Work out the finished part from the listing and answer in its coordinate system (mm). Face numbers are marked on the shaded views. A direction names the side the tool comes from. Coordinates: 2 decimals unless noted, no trailing zeros. Loops run counter-clockwise (first coordinate to the right, second up) from the corner with the lowest first, then second, coordinate; pieces in that order, holes last. Notation, with made-up numbers: (6, 79.5) -> (40, 79.5) arc R13 cw to (40, 95.5) -> close; hole circle Ø7 at (-25.5, 15.25). An arc over 180 degrees is marked (long way). Use a Markdown table: item, result.
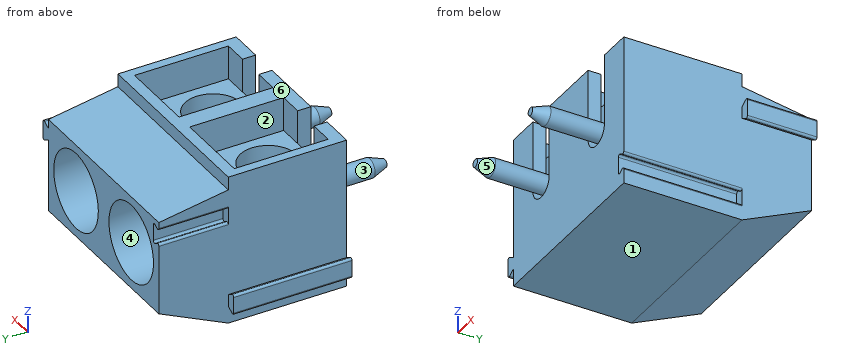
from build123d import *

# Parameters (mm, degrees)
BOSS_EXTRUDE1_DEPTH      = 10.16
SKETCH2_W                = 4.1
SKETCH2_H                = 5
CUT_EXTRUDE1_DEPTH       = 5.8
SKETCH3_W                = 4.1
SKETCH3_H                = 5
CUT_EXTRUDE2_DEPTH       = 5.8
CUT_EXTRUDE3_DEPTH       = 1
CUT_EXTRUDE4_DEPTH       = 1
BOSS_EXTRUDE2_DEPTH      = 2
BOSS_EXTRUDE2_DEPTH_BACK = 2
SKETCH6_W                = 4.1
SKETCH6_H                = 4.7
SKETCH6_R                = 1.5
BOSS_EXTRUDE3_DEPTH      = 2
BOSS_EXTRUDE3_DEPTH_BACK = 2
SKETCH7_W                = 4.1
SKETCH7_H                = 4.7
SKETCH7_R                = 1.5
SKETCH10_W               = 2.05
SKETCH10_H               = 2
SKETCH11_W               = 2.05
SKETCH11_H               = 2
BOSS_EXTRUDE4_DEPTH      = 6.3
CUT_EXTRUDE5_DEPTH       = 6.3
CUT_EXTRUDE6_DEPTH       = 3.7
BOSS_EXTRUDE5_DEPTH      = 3.7


with BuildPart() as part:
    # Sketch1 → Boss-Extrude1 (new body)
    with BuildSketch(Plane(origin=(0, 0, 0), x_dir=(0, 0, -1), z_dir=(1, 0, 0))):
        Polygon((-8, 0), (0, 0), (0, 6.3), (-1.7, 10), (-6.7, 10), (-7.3, 6.3), (-8, 6.3), align=None)
    extrude(amount=BOSS_EXTRUDE1_DEPTH)

    # Sketch2 → Cut-Extrude1 (cut)
    with BuildSketch(Plane.XY.offset(8)):
        with Locations((2.54, 3.2)):
            Rectangle(SKETCH2_W, SKETCH2_H)
    extrude(amount=-CUT_EXTRUDE1_DEPTH, mode=Mode.SUBTRACT)

    # Sketch3 → Cut-Extrude2 (cut)
    with BuildSketch(Plane.XY.offset(8)):
        with Locations((7.62, 3.2)):
            Rectangle(SKETCH3_W, SKETCH3_H)
    extrude(amount=-CUT_EXTRUDE2_DEPTH, mode=Mode.SUBTRACT)

    # Sketch4 → Cut-Extrude3 (cut)
    with BuildSketch(Plane(origin=(0, 0, 0), x_dir=(-1, 0, 0), z_dir=(0, 1, 0))):
        with BuildLine():
            Line((-1.79, 4.2), (-1.79, 8))
            Line((-1.79, 8), (-3.29, 8))
            Line((-3.29, 8), (-3.29, 4.2))
            ThreePointArc((-3.29, 4.2), (-2.54, 3.45), (-1.79, 4.2))
        make_face()
    extrude(amount=CUT_EXTRUDE3_DEPTH, mode=Mode.SUBTRACT)

    # Sketch5 → Cut-Extrude4 (cut)
    with BuildSketch(Plane(origin=(0, 0, 0), x_dir=(-1, 0, 0), z_dir=(0, 1, 0))):
        with BuildLine():
            Line((-6.87, 4.2), (-6.87, 8))
            Line((-6.87, 8), (-8.37, 8))
            Line((-8.37, 8), (-8.37, 4.2))
            ThreePointArc((-8.37, 4.2), (-7.62, 3.45), (-6.87, 4.2))
        make_face()
    extrude(amount=CUT_EXTRUDE4_DEPTH, mode=Mode.SUBTRACT)

    # Sketch6 → Boss-Extrude2 (add, two sides: drawn at the far end of the back side and taken through both)
    with BuildSketch(Plane.XY.offset(4.2).offset(-BOSS_EXTRUDE2_DEPTH_BACK)):
        with Locations((2.54, 3.05)):
            Rectangle(SKETCH6_W, SKETCH6_H)
        with Locations((2.54, 2.7)):
            Circle(SKETCH6_R, mode=Mode.SUBTRACT)
    extrude(amount=BOSS_EXTRUDE2_DEPTH + BOSS_EXTRUDE2_DEPTH_BACK)

    # Sketch7 → Boss-Extrude3 (add, two sides: drawn at the far end of the back side and taken through both)
    with BuildSketch(Plane.XY.offset(4.2).offset(-BOSS_EXTRUDE3_DEPTH_BACK)):
        with Locations((7.62, 3.05)):
            Rectangle(SKETCH7_W, SKETCH7_H)
        with Locations((7.62, 2.7)):
            Circle(SKETCH7_R, mode=Mode.SUBTRACT)
    extrude(amount=BOSS_EXTRUDE3_DEPTH + BOSS_EXTRUDE3_DEPTH_BACK)

    # Sketch8 → Revolve1 (revolve)
    with BuildSketch(Plane.XY.offset(4.2), mode=Mode.PRIVATE) as revolve1_sk:
        Polygon((2.54, 0.7), (3.04, 0.7), (3.04, -2.7), (2.748823813, -3.5), (2.54, -3.5), align=None)
    revolve(revolve1_sk.sketch.rotate(Axis((2.54, -3.5, 4.2), (0, 1, 0)), 270), axis=Axis((2.54, -3.5, 4.2), (0, 1, 0)))

    # Sketch9 → Revolve2 (revolve)
    with BuildSketch(Plane.XY.offset(4.2), mode=Mode.PRIVATE) as revolve2_sk:
        Polygon((7.62, 0.7), (8.12, 0.7), (8.12, -2.7), (7.828823813, -3.5), (7.62, -3.5), align=None)
    revolve(revolve2_sk.sketch.rotate(Axis((7.62, -3.5, 4.2), (0, 1, 0)), 270), axis=Axis((7.62, -3.5, 4.2), (0, 1, 0)))

    # Sketch10 → Cut-Revolve1 (revolve, cut)
    with BuildSketch(Plane.XY.offset(4.2), mode=Mode.PRIVATE) as cut_revolve1_sk:
        with Locations((3.565, 9)):
            Rectangle(SKETCH10_W, SKETCH10_H)
    revolve(cut_revolve1_sk.sketch.rotate(Axis((2.54, 8, 4.2), (0, 1, 0)), 270), axis=Axis((2.54, 8, 4.2), (0, 1, 0)), mode=Mode.SUBTRACT)

    # Sketch11 → Cut-Revolve2 (revolve, cut)
    with BuildSketch(Plane.XY.offset(4.2), mode=Mode.PRIVATE) as cut_revolve2_sk:
        with Locations((8.645, 9)):
            Rectangle(SKETCH11_W, SKETCH11_H)
    revolve(cut_revolve2_sk.sketch.rotate(Axis((7.62, 8, 4.2), (0, 1, 0)), 270), axis=Axis((7.62, 8, 4.2), (0, 1, 0)), mode=Mode.SUBTRACT)

    # Sketch12 → Boss-Extrude4 (add)
    with BuildSketch(Plane(origin=(0, 0, 0), x_dir=(-1, 0, 0), z_dir=(0, 1, 0))):
        with BuildLine():
            Line((0.35, 1.767072594), (0, 1.565))
            Line((0, 1.565), (0, 0.935))
            Line((0, 0.935), (0.35, 0.732927406))
            ThreePointArc((0.35, 0.732927406), (0.45, 0.732927406), (0.5, 0.819529946))
            Line((0.5, 0.819529946), (0.5, 1.680470054))
            ThreePointArc((0.5, 1.680470054), (0.45, 1.767072594), (0.35, 1.767072594))
        make_face()
    extrude(amount=BOSS_EXTRUDE4_DEPTH)

    # Sketch13 → Cut-Extrude5 (cut)
    with BuildSketch(Plane(origin=(0, 0, 0), x_dir=(-1, 0, 0), z_dir=(0, 1, 0))):
        with BuildLine():
            Line((-9.81, 1.767072594), (-10.01, 1.65160254))
            ThreePointArc((-10.01, 1.65160254), (-10.11, 1.65160254), (-10.16, 1.738205081))
            Line((-10.16, 1.738205081), (-10.16, 1.865))
            Line((-10.16, 1.865), (-10.46, 1.865))
            Line((-10.46, 1.865), (-10.46, 0.635))
            Line((-10.46, 0.635), (-10.16, 0.635))
            Line((-10.16, 0.635), (-10.16, 0.761794919))
            ThreePointArc((-10.16, 0.761794919), (-10.11, 0.84839746), (-10.01, 0.84839746))
            Line((-10.01, 0.84839746), (-9.81, 0.732927406))
            ThreePointArc((-9.81, 0.732927406), (-9.71, 0.732927406), (-9.66, 0.819529946))
            Line((-9.66, 0.819529946), (-9.66, 1.680470054))
            ThreePointArc((-9.66, 1.680470054), (-9.71, 1.767072594), (-9.81, 1.767072594))
        make_face()
    extrude(amount=CUT_EXTRUDE5_DEPTH, mode=Mode.SUBTRACT)

    # Sketch14 → Cut-Extrude6 (cut)
    with BuildSketch(Plane(origin=(0, 10, 0), x_dir=(-1, 0, 0), z_dir=(0, 1, 0))):
        with BuildLine():
            Line((0.2, 6.4), (0, 6.4))
            Line((0, 6.4), (0, 6.373205081))
            ThreePointArc((0, 6.373205081), (-0.05, 6.28660254), (-0.15, 6.28660254))
            Line((-0.15, 6.28660254), (-0.35, 6.402072594))
            ThreePointArc((-0.35, 6.402072594), (-0.45, 6.402072594), (-0.5, 6.315470054))
            Line((-0.5, 6.315470054), (-0.5, 5.454529946))
            ThreePointArc((-0.5, 5.454529946), (-0.45, 5.367927406), (-0.35, 5.367927406))
            Line((-0.35, 5.367927406), (-0.15, 5.48339746))
            ThreePointArc((-0.15, 5.48339746), (-0.05, 5.48339746), (0, 5.396794919))
            Line((0, 5.396794919), (0, 5.37))
            Line((0, 5.37), (0.2, 5.37))
            Line((0.2, 5.37), (0.2, 6.4))
        make_face()
    extrude(amount=-CUT_EXTRUDE6_DEPTH, mode=Mode.SUBTRACT)

    # Sketch15 → Boss-Extrude5 (add)
    with BuildSketch(Plane(origin=(0, 10, 0), x_dir=(-1, 0, 0), z_dir=(0, 1, 0))):
        with BuildLine():
            Line((-10.16, 6.2), (-10.51, 6.402072594))
            ThreePointArc((-10.51, 6.402072594), (-10.61, 6.402072594), (-10.66, 6.315470054))
            Line((-10.66, 6.315470054), (-10.66, 5.454529946))
            ThreePointArc((-10.66, 5.454529946), (-10.61, 5.367927406), (-10.51, 5.367927406))
            Line((-10.51, 5.367927406), (-10.16, 5.57))
            Line((-10.16, 5.57), (-10.16, 6.2))
        make_face()
    extrude(amount=-BOSS_EXTRUDE5_DEPTH)


solid = part.part
Q1. Determine the mould class of the marked faces 5 and 6 for opening direction X: pulls with the +X half, pulls with the -X half, needs draft (parallel to the pull), parting line crosses it, or undercut.
Solved:
| item | result |
|---|---|
| face 5 | undercut |
| face 6 | needs draft |
Q2. Given pin 1 Ø4 at (y, z) = (8, 3) entering from +X; pin 2 Ø3.5 at (x, y) = (2.54, 2.7) entering from +Z; pin 3 Ø2 at (x, z) = (1.5, 5.5) entering from -Y, each flat-ended and moving along its own axis, determine where each tip first touches the part or whether it passes through.
Solved:
| item | result |
|---|---|
| pin 1 | x = 10.16 |
| pin 2 | z = 6.2 |
| pin 3 | y = 0 |
Q3. Section B-B on x = 2.54 is taken. Determine the outline of the cut face in (y, z).
Solved:
| item | result |
|---|---|
| outline | (-3.5, 3.99) -> (-2.7, 3.7) -> (0.7, 3.7) -> (0.7, 3.45) -> (0, 3.45) -> (0, 0) -> (6.3, 0) -> (10, 1.7) -> (10, 2.15) -> (8, 2.15) -> (8, 6.25) -> (10, 6.25) -> (10, 6.7) -> (6.3, 7.3) -> (6.3, 8) -> (5.7, 8) -> (5.7, 2.2) -> (5.4, 2.2) -> (5.4, 6.2) -> (4.2, 6.2) -> (4.2, 2.2) -> (1.2, 2.2) -> (1.2, 6.2) -> (0.7, 6.2) -> (0.7, 4.7) -> (-2.7, 4.7) -> (-3.5, 4.41) -> close |
Q4. Section C-C on z = 6 is taken. State how many separate pieces and enclosed holes the cut face has, and give its area (3 significant figures).
Solved:
| item | result |
|---|---|
| separate pieces | 1 |
| enclosed holes | 4 |
| area | 75.1 mm² |
Q5. Section D-D on y = 9 is taken. Determine the outline of the cut face in (x, z), and give its area (3 significant figures).
Solved:
| item | result |
|---|---|
| outline | (0, 1.24) -> (10.16, 1.24) -> (10.16, 5.57) -> (10.51, 5.37) arc R0.1 ccw to (10.66, 5.45) -> (10.66, 6.32) arc R0.1 ccw to (10.51, 6.4) -> (10.16, 6.2) -> (10.16, 6.86) -> (0, 6.86) -> (0, 6.37) arc R0.1 ccw to (0.15, 6.29) -> (0.35, 6.4) arc R0.1 cw to (0.5, 6.32) -> (0.5, 5.45) arc R0.1 cw to (0.35, 5.37) -> (0.15, 5.48) arc R0.1 ccw to (0, 5.4) -> close; hole circle Ø4.1 at (2.54, 4.2); hole circle Ø4.1 at (7.62, 4.2) |
| area | 30.7 mm² |
Q6. Consider line 1 (X direction, y = 9.05, z = 4.2); line 2 (Y direction, x = 7.62, z = 3.6); line 3 (Y direction, x = 6.5, z = 5.5). Determine where each line is inside the solid, lowest interval first. Write a range as [from, to].
Solved:
| item | result |
|---|---|
| line 1 | [0, 0.49], [4.59, 5.57], [9.67, 10.16] |
| line 2 | [0.7, 1.2], [4.2, 5.4], [5.7, 8] |
| line 3 | [0, 1.7], [3.7, 5.4], [5.7, 8] |
Q7. For the marked faces 1, 2, 3 and 4, determine the directions among +Z, -Z, +X, -X, +Y, -Y from which every point of the face is accessible in a straight line to the end or side of a thin tool.
Solved:
| item | result |
|---|---|
| face 1 | -Z, +X, -X, +Y, -Y |
| face 2 | +Z |
| face 3 | -Y |
| face 4 | +Y |
